For this review, take the finished solid that the model builds, in its own axes (mm). Face numbers are marked on the shaded views. A direction names the side the tool comes from. Coordinates: 2 decimals unless noted, no trailing zeros. Loops run counter-clockwise (first coordinate to the right, second up) from the corner with the lowest first, then second, coordinate; pieces in that order, holes last. Notation, with made-up numbers: (84, -30) - (135, -30) arc R8 ccw to (135, -26) - close; hole circle Ø5 at (22.25, 48.25). An arc over 180 degrees is marked (long way). Use one line per item in the form item = value. Start each with the question number.
1. Machinability: for the marked faces 4, 5, 6 and 7, which of the approach directions +Z, -Z, +X, -X, +Y, -Y give a long, thin tool a straight path to every point of the face, cutting with its end or side? Answer none if there is none.
2. For pin 1 Ø7 at (x, z) = (-49.5, -6) entering from -Y; pin 2 Ø4 at (y, z) = (-51.5, -3) entering from +X; pin 3 Ø1.5 at (y, z) = (-57.5, -7.5) entering from -X; pin 4 Ø8 at (x, z) = (-68, -1.5) entering from +Y, all flat-tipped, find the tip position at first contact; note any pin that passes through.
3. Add section A-A on z = 2.5. Give the boundary of the cut face in (x, y), and give its area (3 significant figures).
4. Add section C-C on x = -65. Give the boundary of the cut face in (y, z).
5. Add section D-D on z = -1. Give the boundary of the cut face in (x, y).
6. Add section B-B on y = -4. Give the boundary of the cut face in (x, z).
7. Draft analysis for pull direction Z (two halves, no side actions). For the marked faces 1, 2 and 3, state which applies: +Z half, -Z half, draft (parallel to the pull), parting line (faces both ways), or undercut.
8. To check wall thickness, follow probe 1 along Z at (x, y) = (-65, -24); probe 2 along Y at (x, z) = (-52, -7.75); probe 3 along X at (y, z) = (-34.5, 0.5). State the ranges of each line that lie inside material, in increasing order.
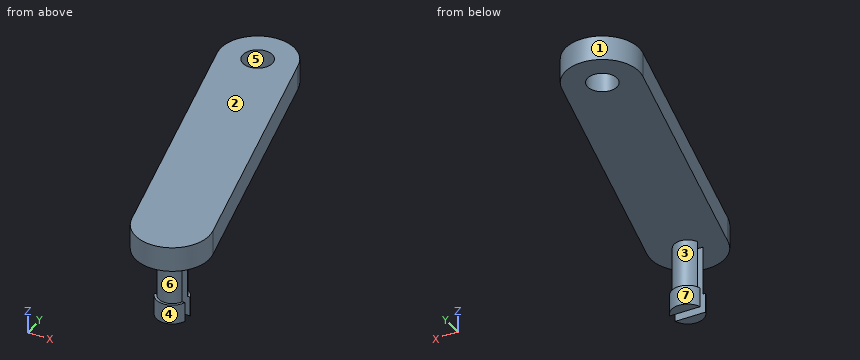
```python
from build123d import *

# Parameters (mm, degrees)
BOSS_EXTRU_1_DEPTH      = 5
ESQUISSE2_R             = 2.75
BOSS_EXTRU_2_DEPTH      = 15
ESQUISSE4_R             = 3.25
BOSS_EXTRU_3_DEPTH      = 4
ESQUISSE5_W             = 10
ESQUISSE5_H             = 2
ENL_V_MAT_EXTRU_2_DEPTH = 14
ESQUISSE6_R             = 3
ENL_V_MAT_EXTRU_3_DEPTH = 14


with BuildPart() as part:
    # Esquisse1 → Boss.-Extru.1 (new body)
    with BuildSketch(Plane.XY):
        with BuildLine():
            Line((-56.704090657, -2.262269623), (-43.729037177, -56.738392716))
            ThreePointArc((-43.729037177, -56.738392716), (-49.287216143, -65.772032435), (-58.320855862, -60.213853469))
            Line((-58.320855862, -60.213853469), (-71.295909343, -5.737730377))
            ThreePointArc((-71.295909343, -5.737730377), (-65.737730377, 3.295909343), (-56.704090657, -2.262269623))
        make_face()
    extrude(amount=BOSS_EXTRU_1_DEPTH)

    # Esquisse2 → Boss.-Extru.2 (add)
    with BuildSketch(Plane.XY.offset(5)):
        with Locations((-51.024946519, -58.476123092)):
            Circle(ESQUISSE2_R)
    extrude(amount=-BOSS_EXTRU_2_DEPTH)

    # Esquisse4 → Boss.-Extru.3 (add)
    with BuildSketch(Plane(origin=(0, 0, -10), x_dir=(-1, 0, 0), z_dir=(0, 0, -1))):
        with Locations((51.024946519, -58.476123092)):
            Circle(ESQUISSE4_R)
    extrude(amount=BOSS_EXTRU_3_DEPTH)

    # Esquisse5 → Enlèv. mat.-Extru.2 (cut)
    with BuildSketch(Plane(origin=(0, 0, -14), x_dir=(-1, 0, 0), z_dir=(0, 0, -1))):
        with Locations((51.024946519, -58.476123092)):
            Rectangle(ESQUISSE5_W, ESQUISSE5_H)
    extrude(amount=-ENL_V_MAT_EXTRU_2_DEPTH, mode=Mode.SUBTRACT)

    # Esquisse6 → Enlèv. mat.-Extru.3 (cut)
    with BuildSketch(Plane.XY.offset(5)):
        with Locations((-64, -4)):
            Circle(ESQUISSE6_R)
    extrude(amount=-ENL_V_MAT_EXTRU_3_DEPTH, mode=Mode.SUBTRACT)


solid = part.part
```
Conclusion:
q1.face_4 = -Z, -Y
q1.face_5 = +Z, -Z
q1.face_6 = -Y
q1.face_7 = -Z, +Y
q2.pin_1 = -61.23
q2.pin_2 = through
q2.pin_3 = -53.59
q2.pin_4 = 3.49
q3.outline = (-71.3, -5.74) - (-58.32, -60.21) arc R7.5 ccw to (-43.73, -56.74) - (-56.7, -2.26) arc R7.5 ccw to start; hole circle Ø6 at (-64, -4)
q3.area = 988 mm^2
q4.outline = (-32.17, 0) - (-6.83, 0) - (-6.83, 5) - (-32.17, 5) - close; (-1.17, 0) - (3.43, 0) - (3.43, 5) - (-1.17, 5) - close
q5.outline = (-53.59, -59.48) arc R2.75 ccw to (-48.46, -59.48) - close; (-53.59, -57.48) - (-48.46, -57.48) arc R2.75 ccw to start
q6.outline = (-71.5, 0) - (-67, 0) - (-67, 5) - (-71.5, 5) - close; (-61, 0) - (-56.29, 0) - (-56.29, 5) - (-61, 5) - close
q7.face_1 = draft
q7.face_2 = +Z half
q7.face_3 = undercut
q8.probe_1 = 0 to 5
q8.probe_2 = -61.05 to -59.48, -57.48 to -55.9
q8.probe_3 = -64.45 to -49.03
